CAD build for the part. Positions are in the model's coordinates, mm. Face numbers are marked on the shaded views. A direction names the side the tool comes from. Coordinates: 2 decimals unless noted, no trailing zeros. Loops run counter-clockwise (first coordinate to the right, second up) from the corner with the lowest first, then second, coordinate; pieces in that order, holes last. Notation, with made-up numbers: (69.25, 74.25) -> (90.25, 74.25) arc R4 cw to (90.25, 78.25) -> close; hole circle Ø3 at (40.5, 7.5). An arc over 180 degrees is marked (long way). Write item = value, one per line. Start each with the question number.
(1) Band-saw the part on D-D (z = 17.5). Write the cut outline in (x, y).
(2) Band-saw the part on C-C (z = 0.25). Write the cut outline in (x, y), and give its area (3 significant figures).
(3) Tool access for the marked faces 1 and 2: list every direction of +Z, -Z, +X, -X, +Y, -Y with a clear straight run to the whole face (end or side of a thin tool).
(4) Flat gauge pins, fed straight in: P1, Ø1.5, axis at x = -2, z = 0.5, coming from the +Y side; P2, Ø1.1, axis at x = 0, y = -1, coming from the +Z side; P3, Ø1, axis at x = -2, z = 10, coming from the +Y side. Where does each tip first touch, or does it go through?
(5) Drill centre lines: line 1 (Y direction, x = 0, z = 15.75); line 2 (Z direction, x = 1.25, y = -3); line 3 (Y direction, x = -1.5, z = 16). Where is each one in solid material? Low to high. Write a range as from..to.
(6) Pull direction Y, two halves, no side cores. Call the marked faces 3, 4 and 5: +Y half, -Y half, draft (parallel to the pull), parting line (faces both ways), or undercut.
(7) Band-saw the part on A-A (x = 0). Write the cut outline in (y, z).
```python
from build123d import *

# Parameters (mm, degrees)
SKETCH_R     = 3.75
PAD_DEPTH    = 20
SKETCH001_R  = 1.85
POCKET_DEPTH = 9
SKETCH002_R  = 2.1
PAD001_DEPTH = 5
FILLET_R     = 1


with BuildPart() as part:
    # Sketch → Pad (new body)
    with BuildSketch(Plane.XY):
        Circle(SKETCH_R)
    extrude(amount=PAD_DEPTH)

    # Sketch001 (on Face3 of Pad) → Pocket (cut)
    with BuildSketch(Plane.XY.offset(20)):
        Circle(SKETCH001_R)
    extrude(amount=-POCKET_DEPTH, mode=Mode.SUBTRACT)

    # Sketch002 (on Face2 of Pocket) → Pad001 (join)
    with BuildSketch(Plane(origin=(0, 0, 0), x_dir=(1, 0, 0), z_dir=(0, 0, -1))):
        Circle(SKETCH002_R)
    extrude(amount=PAD001_DEPTH)

    # Fillet
    fillet_edges = [part.edges().sort_by_distance(p)[0] for p in [
        (-2.1, 0, -5),
    ]]
    fillet(fillet_edges, radius=FILLET_R)


solid = part.part
```
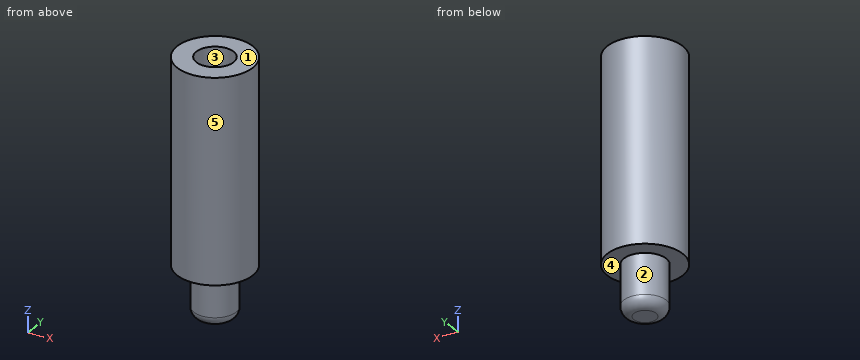
Findings below:
q1.outline = circle Ø7.5 at (0, 0); hole circle Ø3.7 at (0, 0)
q2.outline = circle Ø7.5 at (0, 0)
q2.area = 44.2 mm²
q3.face_1 = +Z, +X, -X, +Y, -Y
q3.face_2 = -Z
q4.P1 = 3.54
q4.P2 = 11
q4.P3 = 3.44
q5.line_1 = -3.75..-1.85, 1.85..3.75
q5.line_2 = 0..20
q5.line_3 = -3.44..-1.08, 1.08..3.44
q6.face_3 = undercut
q6.face_4 = draft
q6.face_5 = parting line
q7.outline = (-3.75, 0) -> (-2.1, 0) -> (-2.1, -4) arc R1 ccw to (-1.1, -5) -> (1.1, -5) arc R1 ccw to (2.1, -4) -> (2.1, 0) -> (3.75, 0) -> (3.75, 20) -> (1.85, 20) -> (1.85, 11) -> (-1.85, 11) -> (-1.85, 20) -> (-3.75, 20) -> close
